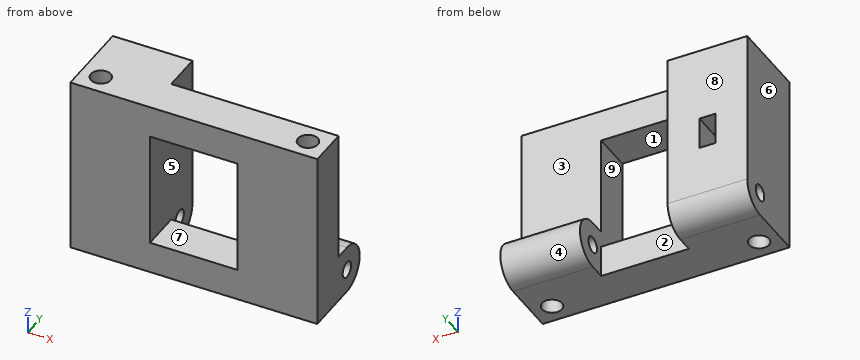
Autodesk Inventor part; units mm, degrees
ref_plane "YZ Plane" through (0, 0, 0) normal (1, 0, 0) x (0, 1, 0)
ref_plane "XZ Plane" through (0, 0, 0) normal (0, 1, 0) x (-1, 0, 0)
ref_plane "XY Plane" through (0, 0, 0) normal (0, 0, 1) x (1, 0, 0)
sketch "Sketch1" plane through (0, 0, 0) normal (0, 1, 0) x (-1, 0, 0)
  line L0 (0, 0) -> (0, -22.5)
  line L1 (0, -22.5) -> (31, -22.5)
  line L2 (31, -22.5) -> (31, 0)
  line L3 (31, 0) -> (0, 0)
  dimension "d0" = 22.5
  dimension "d1" = 31
extrude "Extrusion1" add sketch "Sketch1" along normal blind 5
sketch "Sketch2" plane through (-31, 0, 0) normal (0, 0, 1) x (1, 0, 0)
  line L0 (0, 0) -> (31, 0)
  line L1 (31, 0) -> (31, 5)
  line L2 (0, 5) -> (31, 5)
  line L3 (0, 0) -> (0, 5)
  line L4 (0, 0) -> (0, 5)
  line L5 (0, 2.5) -> (2.5, 2.5)
  circle A0 centre (2.5, 2.5) radius 1.25
  dimension "d4" = 2.5
  dimension "d5" = 2.5
extrude "Extrusion2" cut sketch "Sketch2" against normal up to next contours A0
ref_plane "Work Plane1" through (-15.5, 0, 0) normal (1, 0, 0) x (0, 0, -1)
mirror "Mirror1" about plane through (-15.5, 0, 0) normal (1, 0, 0) of "Extrusion2"
sketch "Sketch3" plane through (0, 5, 0) normal (0, 1, 0) x (1, 0, 0)
  line L0 (0, 0) -> (0, 22.5)
  line L1 (0, 22.5) -> (-31, 22.5)
  line L2 (-31, 22.5) -> (-31, 0)
  line L3 (-31, 0) -> (0, 0)
  line L4 (0, 22.5) -> (-31, 22.5)
  line L5 (-15.5, 22.5) -> (-15.5, 18.5)
  line L6 (-31, 0) -> (0, 0)
  line L7 (-15.5, 0) -> (-15.5, 4)
  line L8 (-21, 18.5) -> (-10, 18.5)
  line L9 (-10, 18.5) -> (-10, 4)
  line L10 (-21, 4) -> (-21, 18.5)
  line L11 (-31, 22.5) -> (-31, 0)
  line L12 (-10, 4) -> (-15.5, 4)
  line L13 (-15.5, 4) -> (-21, 4)
  dimension "d8" = 4
  dimension "d9" = 4
  dimension "d11" = 11
extrude "Extrusion3" cut sketch "Sketch3" against normal up to next contours L13 L10 L8 L9 L12
sketch "Sketch4" plane through (0, 0, 0) normal (1, 0, 0) x (0, 0, -1)
  line L0 (0, 0) -> (22.5, 0)
  line L1 (22.5, 0) -> (22.5, 5)
  line L2 (0, 5) -> (22.5, 5)
  line L3 (0, 0) -> (0, 5)
  line L4 (0, 5) -> (22.5, 5)
  line L5 (22.5, 0) -> (22.5, 5)
  line L6 (22.5, 5) -> (22.5, 7)
  line L7 (22.5, 7) -> (19.5, 7)
  arc A0 (22.5, 7) -> (16.5, 7) centre (19.5, 7) ccw
  line L8 (16.5, 7) -> (16.5, 5)
  circle A1 centre (19.5, 7) radius 1
  dimension "d21" = 2
  dimension "d22" = 3
  dimension "d23" = 2
extrude "Extrusion4" add sketch "Sketch4" against normal blind 10 contours L2 L8 A0 L6
ref_plane "Work Plane2" through (-15.5, 0, -22.5) normal (-1, 0, 0) x (0, 0, 1)
mirror "Mirror2" about plane through (-15.5, 0, -22.5) normal (-1, 0, 0) of "Extrusion4"
sketch "Sketch6" plane through (-31, 0, -22.5) normal (-1, 0, 0) x (0, 0, 1)
  circle A0 centre (3, 7) radius 1
  line L0 (0, 0) -> (22.5, 0)
  line L1 (22.5, 0) -> (22.5, 5)
  line L2 (6, 5) -> (22.5, 5)
  line L3 (6, 7) -> (6, 5)
  arc A1 (6, 7) -> (0, 7) centre (3, 7) ccw
  line L4 (0, 0) -> (0, 7)
  arc A2 (6, 7) -> (0, 7) centre (3, 7) ccw
  line L5 (3, 10) -> (22.5, 10)
  line L6 (6, 5) -> (22.5, 5)
  line L7 (22.5, 5) -> (22.5, 10)
extrude "Extrusion6" add sketch "Sketch6" against normal up to surface (10 mm away) contours L2 L3 A1 L5 L7
sketch "Sketch7" plane through (-31, 10, 0) normal (0, 1, 0) x (1, 0, 0)
  line L0 (10, 19.5) -> (10, 0)
  line L1 (10, 19.5) -> (0, 19.5)
  line L2 (0, 0) -> (0, 19.5)
  line L3 (0, 0) -> (10, 0)
  line L4 (6, 13.25) -> (4, 13.25)
  line L5 (4, 13.25) -> (4, 9.25)
  line L6 (4, 9.25) -> (6, 9.25)
  line L7 (6, 9.25) -> (6, 13.25)
  line L8 (0, 0) -> (0, 19.5)
  line L9 (0, 11.25) -> (4, 11.25)
  line L10 (6, 11.25) -> (10, 11.25)
  line L11 (10, 19.5) -> (10, 0)
  line L12 (0, 22.5) -> (10, 22.5)
  line L13 (5, 22.5) -> (5, 13.25)
  line L14 (5, 9.25) -> (5, 0)
  point P0 (31, 0)
  dimension "d28" = 2
  dimension "d29" = 4
extrude "Extrusion7" cut sketch "Sketch7" against normal blind 5 contours L7 L6 L5 L4
properties part number "Carriage"
Could you check a few things on this model? Use its own coordinates, in mm. Face numbers are marked on the shaded views. A direction names the side the tool comes from. Round coordinates to 2 decimals unless told otherwise and drop trailing zeros. Write each loop counter-clockwise with the first axis right and the second up, starting at its lowest first coordinate (ties: lowest second). Pieces come first, ordered by that corner, then holes. Notation, with made-up numbers: M 2,-32 L 22,-32 A26 ccw 22,0 Z; hole C 4.5,54.25 d5. An arc over 180 degrees is marked long. Answer in a Markdown table with one row per item. Add a question column.
Q1. On a 3-axis mill with a long thin cutter (end or side, diameter ignored), from which of +Z, -Z, +X, -X, +Y, -Y can I reach the whole of each face in a straight line? I mean the marked faces 1, 2, 3, 4 and 5. Say none if no direction works.
Q2. Will these pins go through, and if not, where does the flat tip stop? pin 1 Ø8 at (x, z) = (-11.5, -11) entering from +Y; pin 2 Ø1.5 at (x, z) = (-6, -18) entering from +Y; pin 3 Ø1.2 at (y, z) = (7.5, -11) entering from +X.
Q3. Imagine slicing it at A-A (z = -13.75). Please give me the cut outline in (x, y).
Q4. If I drill on line 1 (Y direction, x = -28.5, z = -10.25); line 2 (Z direction, x = -12, y = 3); line 3 (X direction, y = 5.5, z = -12.5), over which ranges is the centre line in solid material (lowest first)? Write a range as from..to.
Q5. Imagine slicing it at C-C (x = -2.5). Please give me the cut outline in (y, z).
Q6. Imagine slicing it at D-D (z = -3.5). Please give me the cut outline in (x, y).
Q7. Imagine slicing it at B-B (y = 2.5). Please give me the cut outline in (x, z), then the cut area to 4 significant figures.
Q8. If we mould it in two halves opening along X, with no side actions, what happens to the marked faces 6, 7, 8 and 9? For each: +X half, -X half, draft (parallel to the pull), parting line (faces both ways), or undercut.
Values:
| question | item | result |
|---|---|---|
| 1 | face 1 | +Y, -Y |
| 1 | face 2 | +Z, -Z, +Y |
| 1 | face 3 | +Z, +X, +Y |
| 1 | face 4 | +X, +Y |
| 1 | face 5 | +Y |
| 2 | pin 1 | y = 5 |
| 2 | pin 2 | y = 9.9 |
| 2 | pin 3 | x = -21 |
| 3 | outline | M -31,0 L -21,0 L -21,10 L -31,10 Z; M -10,0 L 0,0 L 0,5 L -10,5 Z; hole C -28.5,2.5 d2.5; hole C -2.5,2.5 d2.5 |
| 4 | line 1 | 0..1.25, 3.75..10 |
| 4 | line 2 | -22.5..-18.5, -4..0 |
| 4 | line 3 | -31..-27, -25..-21 |
| 5 | outline | M 0,-22.5 L 1.25,-22.5 L 1.25,0 L 0,0 Z; M 3.75,-22.5 L 7,-22.5 A3 ccw 7,-16.5 L 5,-16.5 L 5,0 L 3.75,0 Z; hole C 7,-19.5 d2 |
| 6 | outline | M -31,0 L 0,0 L 0,5 L -21,5 L -21,10 L -31,10 Z; hole C -28.5,2.5 d2.5; hole C -2.5,2.5 d2.5 |
| 7 | outline | M -31,-22.5 L -29.75,-22.5 L -29.75,0 L -31,0 Z; M -27.25,-22.5 L -3.75,-22.5 L -3.75,0 L -27.25,0 Z; M -1.25,-22.5 L 0,-22.5 L 0,0 L -1.25,0 Z; hole M -21,-18.5 L -10,-18.5 L -10,-4 L -21,-4 Z |
| 7 | area | 425.5 mm^2 |
| 8 | face 6 | -X half |
| 8 | face 7 | undercut |
| 8 | face 8 | draft |
| 8 | face 9 | undercut |
